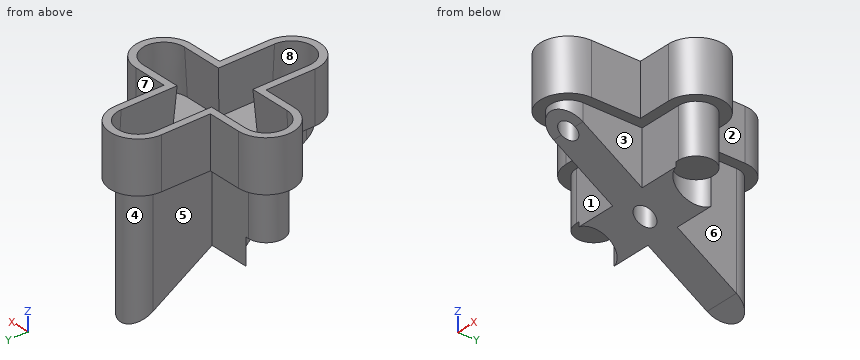
```python
from build123d import *

# Parameters (mm, degrees)
F0_W          = 4.28
F0_H          = 3.44
F0_W_2        = 3.44
F0_H_2        = 5.78
F1_DEPTH      = 12
F3_DEPTH      = 25
F3_DEPTH_BACK = 25
F4_R          = 1.75
F5_DEPTH      = 7.2
F6_R          = 0.9
F7_DEPTH      = 55
F8_R          = 0.9
F10_DEPTH     = 5
F11_R         = 0.8
F12_DEPTH     = 17.001
F14_DEPTH     = 4.5
F14_TAPER     = -3.5


with BuildPart() as f1:
    # F0 (on Top) → F1 (new body)
    with BuildSketch(Plane.XY):
        with Locations((3.86, 0)):
            Rectangle(F0_W, F0_H)
        with BuildLine():
            Line((6, 1.72), (6, -1.72))
            ThreePointArc((6, -1.72), (7.72, 0), (6, 1.72))
        make_face()
        with Locations((0, -4.61)):
            Rectangle(F0_W_2, F0_H_2)
        Rectangle(F0_W_2, F0_H)
        with Locations((-3.86, 0)):
            Rectangle(F0_W, F0_H)
        with BuildLine():
            ThreePointArc((-1.72, -7.5), (0, -9.22), (1.72, -7.5))
            Line((1.72, -7.5), (-1.72, -7.5))
        make_face()
        with Locations((0, 4.61)):
            Rectangle(F0_W_2, F0_H_2)
        with BuildLine():
            ThreePointArc((-6, 1.72), (-7.72, 0), (-6, -1.72))
            Line((-6, -1.72), (-6, 1.72))
        make_face()
        with BuildLine():
            Line((-1.72, 7.5), (1.72, 7.5))
            ThreePointArc((1.72, 7.5), (0, 9.22), (-1.72, 7.5))
        make_face()
    extrude(amount=F1_DEPTH)

    # F2 (on Right) → F3 (cut, two sides)
    with BuildSketch(Plane.YZ) as f3_sk:
        Polygon((-7.5, 0), (7.5, 0), (7.5, 1.0621960754), (-7.5, 10.3255339419), align=None)
        Polygon((7.5, 1.0621960754), (7.5, 0), (9.22, 0), align=None)
        Polygon((-9.22, 0), (-7.5, 0), (-7.5, 10.3255339419), (-9.22, 11.3877300173), align=None)
    extrude(amount=-F3_DEPTH, mode=Mode.SUBTRACT)
    extrude(f3_sk.sketch, amount=F3_DEPTH_BACK, mode=Mode.SUBTRACT)

    # F4 (on Top) → F5 (cut)
    with BuildSketch(Plane.XY):
        with Locations((6, 0)):
            Circle(F4_R)
        with Locations((-6, 0)):
            Circle(F4_R)
    extrude(amount=F5_DEPTH, mode=Mode.SUBTRACT)

    # F6 (on Top) → F7 (cut)
    with BuildSketch(Plane.XY):
        Circle(F6_R)
    extrude(amount=F7_DEPTH, mode=Mode.SUBTRACT)

    # F8 (on face) + F9 (on face) → F10 (join)
    with BuildSketch(Plane.XY.offset(12)):
        with BuildLine():
            Line((1.72, -7.5), (1.72, -1.72))
            Line((1.72, -1.72), (6, -1.72))
            ThreePointArc((6, -1.72), (7.72, 0), (6, 1.72))
            Line((6, 1.72), (1.72, 1.72))
            Line((1.72, 1.72), (1.72, 7.5))
            ThreePointArc((1.72, 7.5), (0, 9.22), (-1.72, 7.5))
            Line((-1.72, 7.5), (-1.72, 1.72))
            Line((-1.72, 1.72), (-6, 1.72))
            ThreePointArc((-6, 1.72), (-7.72, 0), (-6, -1.72))
            Line((-6, -1.72), (-1.72, -1.72))
            Line((-1.72, -1.72), (-1.72, -7.5))
            ThreePointArc((-1.72, -7.5), (0, -9.22), (1.72, -7.5))
        make_face()
        Circle(F8_R, mode=Mode.SUBTRACT)
    with BuildSketch(Plane.XY.offset(12)):
        with BuildLine():
            ThreePointArc((-2.7199999895, -7.5), (0, -10.2199999895), (2.7199999895, -7.5))
            Line((2.7199999895, -7.5), (2.7199999895, -2.7199999895))
            Line((2.7199999895, -2.7199999895), (6, -2.7199999895))
            ThreePointArc((6, -2.7199999895), (8.7199999895, 0), (6, 2.7199999895))
            Line((6, 2.7199999895), (2.7199999895, 2.7199999895))
            Line((2.7199999895, 2.7199999895), (2.7199999895, 7.5))
            ThreePointArc((2.7199999895, 7.5), (0, 10.2199999895), (-2.7199999895, 7.5))
            Line((-2.7199999895, 7.5), (-2.7199999895, 2.7199999895))
            Line((-2.7199999895, 2.7199999895), (-6, 2.7199999895))
            ThreePointArc((-6, 2.7199999895), (-8.7199999895, 0), (-6, -2.7199999895))
            Line((-6, -2.7199999895), (-2.7199999895, -2.7199999895))
            Line((-2.7199999895, -2.7199999895), (-2.7199999895, -7.5))
        make_face()
    extrude(amount=F10_DEPTH)

    # F11 (on face) → F12 (cut, through all)
    with BuildSketch(Plane.XY.offset(17)):
        with Locations((0, -7.5)):
            Circle(F11_R)
    extrude(amount=-F12_DEPTH, mode=Mode.SUBTRACT)

    # F13 (on face) → F14 (cut)
    with BuildSketch(Plane.XY.offset(17)):
        with BuildLine():
            Line((2.02, -2.02), (6, -2.02))
            ThreePointArc((6, -2.02), (8.02, 0), (6, 2.02))
            Line((6, 2.02), (2.02, 2.02))
            Line((2.02, 2.02), (2.02, 7.5))
            ThreePointArc((2.02, 7.5), (0, 9.52), (-2.02, 7.5))
            Line((-2.02, 7.5), (-2.02, 2.02))
            Line((-2.02, 2.02), (-6, 2.02))
            ThreePointArc((-6, 2.02), (-8.02, 0), (-6, -2.02))
            Line((-6, -2.02), (-2.02, -2.02))
            Line((-2.02, -2.02), (-2.02, -7.5))
            ThreePointArc((-2.02, -7.5), (0, -9.52), (2.02, -7.5))
            Line((2.02, -7.5), (2.02, -2.02))
        make_face()
    extrude(amount=-F14_DEPTH, taper=F14_TAPER, mode=Mode.SUBTRACT)


solid = f1.part
```
The listing builds one solid part. Answer for the finished solid, in the listing's coordinates (mm). Face numbers are marked on the shaded views. A direction names the side the tool comes from. Coordinates: 2 decimals unless noted, no trailing zeros. Order: outer loops, then holes, each group sorted by start corner. A loop starts at its lowest first (then second) coordinate and runs counter-clockwise, first axis right, second up. Notation, with made-up numbers: M 49,13.5 L 96,13.5 A18 ccw 96,34.5 Z; hole C 37,2 d4. An arc over 180 degrees is marked long. Answer as a JSON object with one key per item and string values. Group by question number.
1. Section B-B on z = 6.5 is taken. Write down the section's boundary in (x, y).
2. Determine the mould class of the marked faces 5, 6, 7 and 8 for opening direction X: released by +X, released by -X, zero draft, split by the parting line, or undercut.
3. A tool of negligible diameter and unlimited length cuts with its end or side. For the marked faces 1, 2, 3 and 4, from which of +Z, -Z, +X, -X, +Y, -Y can it reach the whole face along a straight path? Write none if from no direction.
4. Straight lines are drawn through the part: line 1 (Y direction, x = 0, z = 11.95); line 2 (X direction, y = -7.5, z = 11.65); line 3 (X direction, y = 0, z = 10.75). For each, find the intervals that lie inside material, in ascending order.
5. Flat-ended cylindrical pins translate along their axes: P1, Ø1.5, axis at y = -2, z = 4.5, coming from the -X side; P2, Ø1, axis at y = -1, z = 9, coming from the -X side; P3, Ø3, axis at x = 6, y = -0.5, coming from the -Z side; P4, Ø3.5, axis at x = -3.5, z = 14, coming from the +Y side. Find the tip coordinate at first contact, or state that the pin passes through.
6. Section A-A on x = 0 is taken. Write down the section's boundary in (y, z), then the cut area to 3 significant figures.
7. Section D-D on z = 1.75 is taken. Write down the section's boundary in (x, y), then the cut area to 3 significant figures.
8. Section C-C on z = 8.5 is taken. Write down the section's boundary in (x, y), then the cut area to 3 significant figures.
Values follow:
{
 "1": {"outline": "M -5.68,1.72 A1.75 cw -4.83,-1.31 L 4.83,-1.31 A1.75 cw 5.68,1.72 L 1.72,1.72 L 1.72,7.5 A1.72 ccw -1.72,7.5 L -1.72,1.72 Z; hole C 0,0 d1.8"},
 "2": {"face 5": "released by -X", "face 6": "released by +X", "face 7": "zero draft", "face 8": "undercut"},
 "3": {"face 1": "-Z, -X, -Y", "face 2": "+Z, -Z, +X, +Y", "face 3": "-Z, +X, -Y", "face 4": "-Z, +Y"},
 "4": {"line 1": "-9.22 to -8.3, -6.7 to -0.9, 0.9 to 9.22", "line 2": "-1.72 to -0.8, 0.8 to 1.72", "line 3": "-7.72 to -0.9, 0.9 to 7.72"},
 "5": {"P1": "through", "P2": "x = -7.65", "P3": "z = 6.35", "P4": "y = 9.58"},
 "6": {"outline": "M -10.22,12 L -9.22,12 L -9.22,11.39 L -8.3,10.82 L -8.3,12.5 L -9.8,12.5 L -9.52,17 L -10.22,17 Z; M -6.7,9.83 L -0.9,6.25 L -0.9,12 L 0.9,12 L 0.9,5.14 L 9.22,0 L 9.22,12 L 10.22,12 L 10.22,17 L 9.52,17 L 9.8,12.5 L -6.7,12.5 Z", "area": "117 mm2"},
 "7": {"outline": "M -1.72,6.39 L 1.72,6.39 L 1.72,7.5 A1.72 ccw -1.72,7.5 Z", "area": "8.48 mm2"},
 "8": {"outline": "M -6,-1.72 L -1.72,-1.72 L -1.72,-4.54 L 1.72,-4.54 L 1.72,-1.72 L 6,-1.72 A1.72 ccw 6,1.72 L 1.72,1.72 L 1.72,7.5 A1.72 ccw -1.72,7.5 L -1.72,1.72 L -6,1.72 A1.72 ccw Z; hole C 0,0 d1.8", "area": "82.3 mm2"}
}
